Verification items for the finished model (mm, model axes). A direction names the side the tool comes from. Coordinates: 2 decimals unless noted, no trailing zeros. Order: outer loops, then holes, each group sorted by start corner. A loop starts at its lowest first (then second) coordinate and runs counter-clockwise, first axis right, second up. Notation, with made-up numbers: M 44,74 L 95,74 A25 cw 95,90 Z; hole C -26,-32.75 d4. An arc over 180 degrees is marked long. Return JSON: item names as keys, results as strings. Group by question number.
1. Section check D-D, the plane z = 37. Record the cut outline in (x, y).
2. Section check A-A, the plane y = -5. Record the cut outline in (x, z), plus the area to 3 significant figures.
3. Material ranges on line 1 along Z through (x, y) = (110.5, -1.5); line 2 along Y through (x, z) = (37, 11.75); line 3 along X through (y, z) = (-4, 24.25), recorded low to high.
4. Section check C-C, the plane z = 14.25. Record the cut outline in (x, y), plus the area to 3 significant figures.
5. Gauge pin test, flat ends, axial feed: pin 1 (11.5 mm diameter, centred on x = 42.5, z = 19.5, fed in from +Y); pin 2 (5.5 mm diameter, centred on x = 96.5, y = -4, fed in from -Z); pin 3 (2 mm diameter, centred on x = 109.5, y = -2, fed in from +Z). Record the tip position at first contact, or that the pin passes through.
6. Mould release check, pull along Z, two halves, no side actions. Record for faces 1 (the flat face through (86, -3, 33.989)), 2 (the cylindrical face through (134.764, -8.624, 30.566)), 3 (the cylindrical face through (47.43, -6.55, 27.91)), 4 (the cylindrical face through (35.085, -3.131, 38.267)): +Z half, -Z half, draft (parallel to the pull), parting line (faces both ways), or undercut.
7. Set-up check for faces 5 (the cylindrical face through (47.432, -6.558, 33.246)), 6 (the cylindrical face through (90.51, 2.23, 33.25)), 7 (the flat face through (31.006, -3.131, 26.804)): record each of +Z, -Z, +X, -X, +Y, -Y from which the full face is reachable in a straight line by a thin tool's end or side.
8. Section check B-B, the plane x = 121. Record the cut outline in (y, z), plus the area to 3 significant figures.
```python
from build123d import *

# Parameters (mm, degrees)
F1_DEPTH = 6.35
F2_W     = 6.35
F2_H     = 4.3350251792
F3_DEPTH = 25.4
F4_DEPTH = 63.5
F5_R     = 2.607278221


# Not quite as in the source:
# - a feature names something its author has since deleted; it is built from what else it names


with BuildPart() as f1:
    # F0 (on Front) → F1 (new body)
    with BuildSketch(Plane.XZ):
        with BuildLine():
            ThreePointArc((38.0586988364, 29.6543792382), (40.3399245407, 31.3092753383), (41.2114633723, 33.9894044175))
            ThreePointArc((41.2114633723, 33.9894044175), (34.9686895654, 38.2226770455), (33.345850058, 30.8565916617))
            ThreePointArc((33.345850058, 30.8565916617), (34.8508967595, 29.8049682674), (36.6488133888, 29.4327141456))
            ThreePointArc((36.6488133888, 29.4327141456), (37.3624884645, 29.4880051728), (38.0586988364, 29.6543792382))
        make_face()
        with BuildLine():
            ThreePointArc((36.6488133888, 29.4327141456), (34.8508967595, 29.8049682674), (33.345850058, 30.8565916617))
            Line((33.345850058, 30.8565916617), (28.5997511098, 22.6370067444))
            Line((28.5997511098, 22.6370067444), (36.9340473419, 10.395447725))
            Line((36.9340473419, 10.395447725), (40.5838886152, 13.2587963652))
            Line((40.5838886152, 13.2587963652), (32.8096505039, 23.1684296974))
            Line((32.8096505039, 23.1684296974), (36.6488133888, 29.4327141456))
        make_face()
        Polygon((56.8539685432, 29.6543792382), (41.3639992476, 29.6543792382), (45.8250723122, 23.9679572756), align=None)
        with BuildLine():
            Line((72.0483290742, 33.9894044175), (41.2114633723, 33.9894044175))
            ThreePointArc((41.2114633723, 33.9894044175), (40.3399245407, 31.3092753383), (38.0586988364, 29.6543792382))
            Line((38.0586988364, 29.6543792382), (41.3639992476, 29.6543792382))
            Line((41.3639992476, 29.6543792382), (56.8539685432, 29.6543792382))
            Line((56.8539685432, 29.6543792382), (72.0483290742, 29.6543792382))
            Line((72.0483290742, 29.6543792382), (72.0483290742, 33.9894044175))
        make_face()
    extrude(amount=F1_DEPTH)

    # F2 (on face) → F3 (join)
    with BuildSketch(Plane.YZ.offset(72.0483290742)):
        Polygon((-6.35, 29.6543792382), (-6.35, 33.9894044175), (-9.3679074198, 33.9894044175), (-9.3679074198, 27.1660927683), (3.0179074198, 27.1660927683), (3.0179074198, 33.9894044175), (0, 33.9894044175), (0, 29.6543792382), align=None)
        with Locations((-3.175, 31.8218918279)):
            Rectangle(F2_W, F2_H)
    extrude(amount=-F3_DEPTH)

    # F4 (add): a face of the model
    f4_faces = [f1.faces().sort_by_distance(p)[0] for p in [
        (72.0483290742, -3.175, 30.5777485929),
    ]]
    extrude(f4_faces, amount=F4_DEPTH)

    # F5
    f5_edges = [f1.edges().sort_by_distance(p)[0] for p in [
        (91.098329, 3.017907, 33.989404),
        (91.098329, 3.017907, 27.166093),
        (91.098329, -9.367907, 27.166093),
        (91.098329, -9.367907, 33.989404),
        (135.548329, -3.175, 33.989404),
        (135.548329, -3.175, 27.166093),
        (135.548329, -9.367907, 30.577749),
        (135.548329, 3.017907, 30.577749),
        (46.648329, 3.017907, 30.577749),
        (46.648329, 1.508954, 33.989404),
        (46.648329, 1.508954, 27.166093),
        (46.648329, -7.858954, 33.989404),
        (46.648329, -7.858954, 27.166093),
        (46.648329, -9.367907, 30.577749),
    ]]
    fillet(f5_edges, radius=F5_R)


solid = f1.part
```
Answers follow:
{
 "1": {"outline": "M 33.23,-6.35 L 40.08,-6.35 L 40.08,0 L 33.23,0 Z"},
 "2": {"outline": "M 28.6,22.64 L 36.93,10.4 L 40.58,13.26 L 32.81,23.17 L 36.65,29.43 A4.56 ccw 38.06,29.65 L 41.36,29.65 L 45.83,23.97 L 52.03,27.17 L 132.94,27.17 A2.61 ccw 135.55,29.77 L 135.55,31.38 A2.61 ccw 132.94,33.99 L 41.21,33.99 A4.56 ccw long 33.35,30.86 Z", "area": "806 mm^2"},
 "3": {"line 1": "27.17 to 33.99", "line 2": "-6.35 to 0", "line 3": "29.53 to 33.47, 45.6 to 46.37"},
 "4": {"outline": "M 34.31,-6.35 L 39.81,-6.35 L 39.81,0 L 34.31,0 Z", "area": "34.9 mm^2"},
 "5": {"pin 1": "y = 0", "pin 2": "z = 27.17", "pin 3": "z = 33.99"},
 "6": {"face 1": "+Z half", "face 2": "draft", "face 3": "-Z half", "face 4": "undercut"},
 "7": {"face 5": "+Z, -X, -Y", "face 6": "+Z, +X, -X, +Y", "face 7": "-X, +Y, -Y"},
 "8": {"outline": "M -9.37,29.77 A2.61 ccw -6.76,27.17 L 0.41,27.17 A2.61 ccw 3.02,29.77 L 3.02,31.38 A2.61 ccw 0.41,33.99 L -6.76,33.99 A2.61 ccw -9.37,31.38 Z", "area": "78.7 mm^2"}
}
